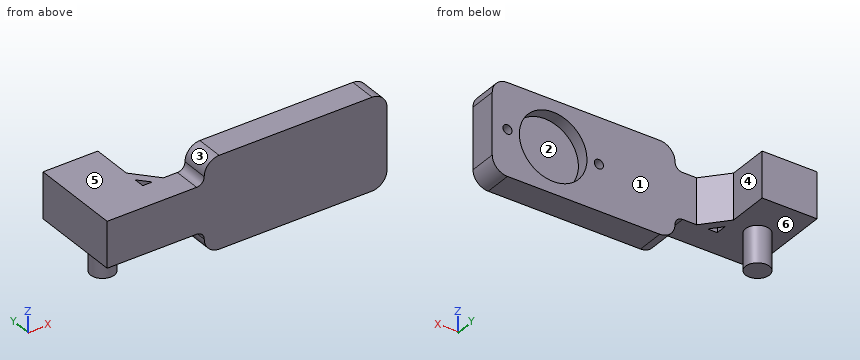
```python
from build123d import *

# Parameters (mm, degrees)
BOSS_EXTRUDE1_DEPTH = 9
SKETCH3_R           = 11.1
SKETCH3_R_2         = 1.5
CUT_EXTRUDE1_DEPTH  = 4
BOSS_EXTRUDE2_DEPTH = 30
BOSS_EXTRUDE4_DEPTH = 15
SKETCH7_R           = 3.9
BOSS_EXTRUDE5_DEPTH = 12


with BuildPart() as part:
    # Sketch1 → Boss-Extrude1 (new body)
    with BuildSketch(Plane(origin=(0, 0, 0), x_dir=(1, 0, 0), z_dir=(0, 1, 0))):
        with BuildLine():
            Line((-25, 11.350947881), (25, 11.350947881))
            ThreePointArc((25, 11.350947881), (28.535533906, 9.886481787), (30, 6.350947881))
            Line((30, 6.350947881), (30, -13.650519031))
            ThreePointArc((30, -13.650519031), (28.578095606, -17.142972586), (25.121107266, -18.649052119))
            Line((25.121107266, -18.649052119), (-25.121107266, -18.649052119))
            ThreePointArc((-25.121107266, -18.649052119), (-28.578095606, -17.142972586), (-30, -13.650519031))
            ThreePointArc((-30, -13.650519031), (-30.731714061, -11.881803874), (-32.49999957, -11.149052119))
            Line((-32.49999957, -11.149052119), (-43.869213178, -11.149052119))
            Line((-43.869213178, -11.149052119), (-43.869213178, 3.850947881))
            Line((-43.869213178, 3.850947881), (-32.5, 3.850947881))
            ThreePointArc((-32.5, 3.850947881), (-30.732233047, 4.583180928), (-30, 6.350947881))
            ThreePointArc((-30, 6.350947881), (-28.535533906, 9.886481787), (-25, 11.350947881))
        make_face()
    extrude(amount=BOSS_EXTRUDE1_DEPTH)

    # Sketch3 → Cut-Extrude1 (cut)
    with BuildSketch(Plane(origin=(0, 9, 0), x_dir=(1, 0, 0), z_dir=(0, 1, 0))):
        with Locations(Location((10, -3.649785575, 0), (0, 0, 270))):
            Circle(SKETCH3_R)
        with Locations(Location((-5, -3.649785575, 0), (0, 0, 270))):
            Circle(SKETCH3_R_2)
        with Locations(Location((25, -3.649785575, 0), (0, 0, 270))):
            Circle(SKETCH3_R_2)
    extrude(amount=-CUT_EXTRUDE1_DEPTH, mode=Mode.SUBTRACT)

    # Sketch2 → Boss-Extrude2 (add)
    with BuildSketch(Plane(origin=(0, 0, 0), x_dir=(1, 0, 0), z_dir=(0, 1, 0))):
        Polygon((-59.869213178, -11.149052119), (-45.869213178, -11.149052119), (-43.869213178, -11.149052119), (-43.869213178, -9.149052119), (-43.869213178, -4.149052119), (-43.869213178, 3.850947881), (-45.869213178, 3.850947881), (-59.869213178, 3.850947881), (-61.869213178, 3.850947881), (-61.869213178, -9.149052119), (-61.869213178, -11.149052119), align=None)
    extrude(amount=BOSS_EXTRUDE2_DEPTH)

    # Sketch6 → Boss-Extrude4 (add)
    with BuildSketch(Plane.XY.offset(11.149052119)):
        Polygon((-43.869213178, 12.558501201), (-40.727008234, 9), (-37.115574999, 9), (-43.869213178, 16.648396589), align=None)
    extrude(amount=-BOSS_EXTRUDE4_DEPTH)

    # Sketch7 → Boss-Extrude5 (add)
    with BuildSketch(Plane(origin=(0, 0, -3.850947881), x_dir=(-1, 0, 0), z_dir=(0, 0, -1))):
        with Locations(Location((52.869213178, 15, 0), (0, 0, 180))):
            Circle(SKETCH7_R)
    extrude(amount=BOSS_EXTRUDE5_DEPTH)


solid = part.part
```
The listing builds one solid part. Answer for the finished solid, in the listing's coordinates (mm). Face numbers are marked on the shaded views. A direction names the side the tool comes from. Round coordinates to 2 decimals unless told otherwise and drop trailing zeros. Loops run counter-clockwise (first coordinate to the right, second up) from the corner with the lowest first, then second, coordinate; pieces in that order, holes last. Notation, with made-up numbers: (77.25, 41) - (108.25, 41) arc R14 ccw to (108.25, 67) - close; hole circle Ø1 at (-10.5, -23). An arc over 180 degrees is marked (long way). Return JSON: item names as keys, results as strings. Group by question number.
1. The part is cut by section A-A on x = 10. Determine the outline of the cut face in (y, z).
2. Consider probe 1 along X at (y, z) = (25.5, 0); probe 2 along X at (y, z) = (6.75, 4.5); probe 3 along Y at (x, z) = (-24, 11). Determine where each line is inside the solid, lowest interval first.
3. The part is cut by section C-C on y = 2.5. Determine the outline of the cut face in (x, z).
4. Which of the six approach directions +Z, -Z, +X, -X, +Y, -Y give full straight-line access (tool end or side, diameter ignored) to the marked faces 4, 5 and 6?
5. Each of these flat-tipped pins is pushed along its axis until it touches: P1, Ø1.8, axis at x = -5, z = 3.65, coming from the +Y side; P2, Ø4, axis at y = 16, z = -4.5, coming from the +X side; P3, Ø15, axis at x = 5.5, z = 8, coming from the +Y side. Where does it stop, or does it pass through?
6. The part is cut by section B-B on z = -3. Determine the outline of the cut face in (x, y).
7. The part is cut by section D-D on z = -9. Determine the outline of the cut face in (x, y).
8. The mould has two halves that part along Z. Classify the marked faces 1, 2 and 3: pulls with the +Z half, pulls with the -Z half, needs draft (parallel to the pull), parting line crosses it, or undercut.
Resolved:
{
 "1": {"outline": "(0, -11.35) - (9, -11.35) - (9, -7.45) - (5, -7.45) - (5, 14.75) - (9, 14.75) - (9, 18.65) - (0, 18.65) - close"},
 "2": {"probe 1": "x = -61.87 to -43.87", "probe 2": "x = -61.87 to -6.24, -3.76 to -1.07, 21.07 to 23.76, 26.24 to 30", "probe 3": "y = 0 to 9"},
 "3": {"outline": "(-61.87, -3.85) - (-32.5, -3.85) arc R2.5 cw to (-30, -6.35) arc R5 ccw to (-25, -11.35) - (25, -11.35) arc R5 ccw to (30, -6.35) - (30, 13.65) arc R5 ccw to (25.12, 18.65) - (-25.12, 18.65) arc R5 ccw to (-30, 13.65) arc R2.5 cw to (-32.5, 11.15) - (-61.87, 11.15) - close"},
 "4": {"face 4": "+Z, -Z, +X, +Y", "face 5": "+Z, -X, +Y, -Y", "face 6": "-Z"},
 "5": {"P1": "stops at y = 5", "P2": "stops at x = -41.63", "P3": "stops at y = 9"},
 "6": {"outline": "(-61.87, 0) - (30, 0) - (30, 9) - (18.89, 9) - (18.89, 5) - (1.11, 5) - (1.11, 9) - (-37.12, 9) - (-43.87, 16.65) - (-43.87, 30) - (-61.87, 30) - close; hole (-43.87, 9) - (-40.73, 9) - (-43.87, 12.56) - close"},
 "7": {"outline": "circle Ø7.8 at (-52.87, 15); (-29.24, 0) - (29.24, 0) - (29.24, 9) - (-29.24, 9) - close"},
 "8": {"face 1": "needs draft", "face 2": "undercut", "face 3": "pulls with the +Z half"}
}
